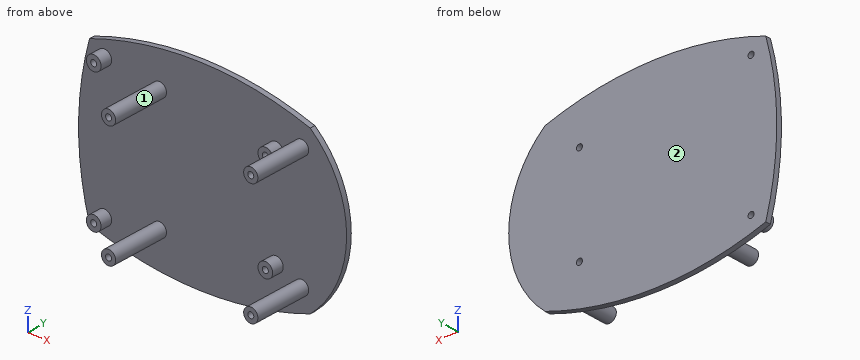
Autodesk Inventor part; units mm, degrees
ref_plane "Arbeitsebene1" through (41.47, 0, -24.5) normal (-0.3949, 0, -0.9187) x (0, -1, 0)
ref_plane "YZ Plane" through (0, 0, 0) normal (1, 0, 0) x (0, 1, 0)
ref_plane "XZ Plane" through (0, 0, 0) normal (0, 1, 0) x (-1, 0, 0)
sketch "Skizze4" plane through (0, 0, 0) normal (0, 1, 0) x (-1, 0, 0)
  arc A0 (45, -32.5) -> (45, 32.5) centre (-70.5152, 0) ccw
  arc A1 (45, 32.5) -> (-45, 32.5) centre (0, -98.75) ccw
  arc A2 (-45, 32.5) -> (-45, -32.5) centre (-16.8442, 0) ccw
  line L0 (49.4848, 0) -> (-59.8442, 0) construction
  circle A3 centre (39, -28) radius 1.225
  circle A4 centre (39, 28) radius 1.225
  circle A5 centre (-31, 20) radius 1.225
  circle A6 centre (-31, -20) radius 1.225
  circle A7 centre (16.53, -24.5) radius 1.225
  circle A8 centre (16.53, 24.5) radius 1.225
  circle A9 centre (-41.47, 24.5) radius 1.225
  circle A10 centre (-41.47, -24.5) radius 1.225
  line L1 (39, 28) -> (39, -28) construction
  line L2 (39, -28) -> (-31, -20) construction
  line L3 (-31, -20) -> (-31, 20) construction
  line L4 (-31, 20) -> (39, 28) construction
  line L5 (16.53, 24.5) -> (16.53, -24.5) construction
  line L6 (16.53, -24.5) -> (-41.47, -24.5) construction
  line L7 (-41.47, -24.5) -> (-41.47, 24.5) construction
  line L8 (-41.47, 24.5) -> (16.53, 24.5) construction
  line L9 (0, -40) -> (0, 40) construction
  circle A11 centre (16.53, -24.5) radius 2.9
  circle A12 centre (-41.47, -24.5) radius 2.9
  circle A13 centre (-41.47, 24.5) radius 2.9
  circle A14 centre (16.53, 24.5) radius 2.9
  line L10 (45, 32.5) -> (45, -32.5) construction
  line L11 (-45, 32.5) -> (-45, -32.5) construction
  arc A15 (-45, -32.5) -> (45, -32.5) centre (0, 98.75) ccw
  circle A16 centre (-31, -20) radius 3
  circle A17 centre (-31, 20) radius 3
  circle A18 centre (39, 28) radius 3
  circle A19 centre (39, -28) radius 3
  point P0 (0, 0)
  point P1 (0, 0)
  dimension "d19" = 2.45
  dimension "d20" = 5.8
  dimension "d28" = 80
  dimension "d30" = 90
  dimension "d31" = 58
  dimension "d32" = 49
  dimension "d33" = 56
  dimension "d34" = 40
  dimension "d35" = 70
  dimension "d36" = 65
  dimension "d37" = 65
  dimension "d38" = 22.47
  dimension "d39" = 120
  dimension "d40" = 6
  dimension "d41" = 2.45
  dimension "d42" = 43
  dimension "d58" = 6
sketch "Skizze3" plane through (0, 0, 0) normal (0, 1, 0) x (-1, 0, 0)
  line L0 (-220.6772, -144.4743) -> (-220.6772, -104.4743)
  line L1 (-220.6772, -104.4743) -> (-150.6772, -96.4743)
  line L2 (-150.6772, -96.4743) -> (-150.6772, -152.4743)
  line L3 (-150.6772, -152.4743) -> (-220.6772, -144.4743)
  line L4 (-173.154, -148.9743) -> (-231.154, -148.9743)
  line L5 (-231.154, -148.9743) -> (-231.154, -99.9743)
  line L6 (-231.154, -99.9743) -> (-173.154, -99.9743)
  line L7 (-173.154, -99.9743) -> (-173.154, -148.9743)
  circle A0 centre (-231.154, -99.9743) radius 1.35
  circle A1 centre (-231.154, -148.9743) radius 1.35
  circle A2 centre (-173.154, -148.9743) radius 1.35
  circle A3 centre (-173.154, -99.9743) radius 1.35
  arc A4 (-234.6505, -110.3469) -> (-234.6486, -138.3994) centre (-219.7787, -124.3722) ccw
  line L8 (-234.6505, -110.3469) -> (-234.6458, -99.4805)
  arc A5 (-231.5992, -96.4365) -> (-234.6458, -99.4805) centre (-231.6005, -99.4818) ccw
  line L9 (-231.5992, -96.4365) -> (-212.1876, -96.4449)
  arc A6 (-178.6836, -89.0505) -> (-212.1876, -96.4449) centre (-176.7514, -177.4047) ccw
  arc A7 (-149.827, -93.1805) -> (-178.6836, -89.0505) centre (-181.982, -214.9715) ccw
  arc A8 (-147.411, -95.6063) -> (-149.827, -93.1805) centre (-150.6924, -96.4584) ccw
  arc A9 (-143.2995, -124.3735) -> (-147.411, -95.6063) centre (-273.1451, -128.2544) ccw
  arc A10 (-147.4215, -153.3903) -> (-143.2995, -124.3735) centre (-273.1519, -120.7284) ccw
  arc A11 (-149.7866, -155.739) -> (-147.4215, -153.3903) centre (-150.6843, -152.4698) ccw
  arc A12 (-178.6402, -159.8288) -> (-149.7866, -155.739) centre (-181.7729, -33.9036) ccw
  arc A13 (-212.2336, -152.5079) -> (-178.6402, -159.8288) centre (-176.9785, -71.4691) ccw
  line L10 (-231.6452, -152.4995) -> (-212.2336, -152.5079)
  arc A14 (-234.6534, -149.2659) -> (-231.6452, -152.4995) centre (-231.6139, -149.4543) ccw
  line L11 (-234.6534, -149.2659) -> (-234.6486, -138.3994)
  line L12 (-240.2208, -124.3735) -> (-143.2995, -124.3735) construction
  line L13 (-177.3977, -89.0907) -> (-177.3977, -159.7918) construction
  point P0 (-177.3977, -124.4413)
extrude "Extrusion1" add sketch "Skizze4" along normal blind 2.2 contours A15 A2 A1 A0 | A7 | A8 | A9 | A10 | A11 | A12 | A13 | A14 | A16 | A17 | A18 | A19
extrude "Extrusion2" add sketch "Skizze4" against normal blind 24 contours A11 | A12 | A13 | A14
extrude "Extrusion3" add sketch "Skizze4" against normal blind 5 contours A16 | A17 | A18 | A19
ref_plane "Arbeitsebene1" through (41.47, 0, -24.5) normal (-0.3949, 0, -0.9187) x (0, -1, 0)
sketch "Skizze6" plane through (41.47, 0, -24.5) normal (-0.3949, 0, -0.9187) x (0, -1, 0)
  line L0 (24, 1.2564) -> (24.1406, 1.5)
  line L1 (24.1406, 1.5) -> (24.1969, 1.5)
  line L2 (24.1969, 1.5) -> (24.3375, 1.2564)
  line L3 (24.3375, 1.2564) -> (24.3937, 1.2564)
  line L4 (24.45, 1.2564) -> (24.45, 1.5487) construction
  line L5 (24.45, 1.5487) -> (23.8875, 1.5487) construction
  line L6 (23.8875, 1.5487) -> (23.8875, 1.2564) construction
  line L7 (23.8875, 1.2564) -> (23.9437, 1.2564) construction
  line L8 (23.9437, 1.2564) -> (24, 1.2564)
  line L9 (24.3937, 1.2564) -> (24.45, 1.2564) construction
  line L10 (24, 1.2564) -> (24.3375, 1.2564) construction
  line L11 (24.1406, 1.5) -> (24.1687, 1.5487) construction
  line L12 (24.1969, 1.5) -> (24.1687, 1.5487) construction
  line L13 (23.8875, 0) -> (24.45, 0) construction
  line L14 (23.8875, 1.2564) -> (23.9437, 1.159) construction
  line L15 (23.9437, 1.159) -> (24, 1.2564) construction
  line L16 (24.3375, 1.2564) -> (24.3937, 1.159) construction
  line L17 (24.3937, 1.159) -> (24.45, 1.2564) construction
  line L18 (24.1687, 1.2564) -> (24.1687, 1.5487) construction
  line L19 (23.9437, 1.159) -> (24.3937, 1.159) construction
  line L20 (23.8875, 0) -> (23.8875, 1.2564) construction
  line L21 (24.45, 0) -> (24.45, 1.2564) construction
  line L22 (-7.98, 0) -> (29.33, 0)
  line L23 (24, 1.225) -> (24, -1.225)
  line L24 (24, 1.2564) -> (24.3375, 1.2564)
  line L25 (-2.5375, 12.6525) -> (-2.3969, 12.8961)
  line L26 (-2.3969, 12.8961) -> (-2.3406, 12.8961)
  line L27 (-2.3406, 12.8961) -> (-2.2, 12.6525)
  line L28 (-2.2, 12.6525) -> (-2.1437, 12.6525)
  line L29 (-2.0875, 12.6525) -> (-2.0875, 12.9448) construction
  line L30 (-2.0875, 12.9448) -> (-2.65, 12.9448) construction
  line L31 (-2.65, 12.9448) -> (-2.65, 12.6525) construction
  line L32 (-2.65, 12.6525) -> (-2.5937, 12.6525) construction
  line L33 (-2.5937, 12.6525) -> (-2.5375, 12.6525)
  line L34 (-2.1437, 12.6525) -> (-2.0875, 12.6525) construction
  line L35 (-2.5375, 12.6525) -> (-2.2, 12.6525) construction
  line L36 (-2.3969, 12.8961) -> (-2.3687, 12.9448) construction
  line L37 (-2.3406, 12.8961) -> (-2.3687, 12.9448) construction
  line L38 (-2.65, 11.3961) -> (-2.0875, 11.3961) construction
  line L39 (-2.65, 12.6525) -> (-2.5937, 12.5551) construction
  line L40 (-2.5937, 12.5551) -> (-2.5375, 12.6525) construction
  line L41 (-2.2, 12.6525) -> (-2.1437, 12.5551) construction
  line L42 (-2.1437, 12.5551) -> (-2.0875, 12.6525) construction
  line L43 (-2.3687, 12.6525) -> (-2.3687, 12.9448) construction
  line L44 (-2.5937, 12.5551) -> (-2.1437, 12.5551) construction
  line L45 (-2.65, 11.3961) -> (-2.65, 12.6525) construction
  line L46 (-2.0875, 11.3961) -> (-2.0875, 12.6525) construction
  line L47 (29.33, 11.3961) -> (-7.98, 11.3961)
  line L48 (-2.5375, 12.6525) -> (-2.2, 12.6525)
  line L49 (-2.2, 10.1711) -> (-2.2, 12.6211)
  dimension "d47" = 60
  dimension "d48" = 3
  dimension "d49" = 0.45
  dimension "d50" = 2.5129
  dimension "d51" = 0.2436
  dimension "d52" = 0.0487
  dimension "d62" = 0
  dimension "d71" = 60
  dimension "d72" = 3
  dimension "d73" = 0.45
  dimension "d74" = 2.5129
  dimension "d75" = 0.2436
  dimension "d76" = 0.0487
  dimension "d82" = 0
equation "\"d53\" = 60deg"
equation "\"d54\" = 3"
equation "\"d55\" = 0.45"
equation "\"d56\" = 2.51288"
equation "\"d57\" = 0.3897"
equation "\"d77\" = 60deg"
equation "\"d78\" = 3"
equation "\"d79\" = 0.45"
equation "\"d80\" = 2.51288"
equation "\"d81\" = 0.3897"
properties part number "_3D-Druck"
The listing builds one solid part. Answer for the finished solid, in the listing's coordinates (mm). Face numbers are marked on the shaded views. Give positions to 0.01 mm unless a question says otherwise; leave off trailing zeros. Loops run counter-clockwise (first coordinate to the right, second up) from the corner with the lowest first, then second, coordinate; pieces in that order, holes last. Notation, with made-up numbers: (87.5, 29.5) - (93.5, 29.5) arc R20 cw to (93.5, 60.5) - close; hole circle Ø10 at (30.25, 76.5). An arc over 180 degrees is marked (long way). Use one line per item in the form item = value.
1. Section C-C on z = -20 is taken. Give the vertices of the cut face in (x, y) (3 decimals).
Calculated:
outline = (-47.806, 0) - (28, 0) - (28, -5) - (29.775, -5) - (29.775, 2.2) - (-47.806, 2.2) - close; (32.225, -5) - (34, -5) - (34, 0) - (54.91, 0) - (54.91, 2.2) - (32.225, 2.2) - close
2. Section B-B on x = -39 is taken. Give the vertices of the cut face in (y, z) (3 decimals).
Calculated:
outline = (-5, -31) - (0, -31) - (0, -34.406) - (2.2, -34.406) - (2.2, -29.225) - (-5, -29.225) - close; (-5, -26.775) - (2.2, -26.775) - (2.2, 26.775) - (-5, 26.775) - (-5, 25) - (0, 25) - (0, -25) - (-5, -25) - close; (-5, 29.225) - (2.2, 29.225) - (2.2, 34.406) - (0, 34.406) - (0, 31) - (-5, 31) - close
3. Section A-A on y = -19.75 is taken. Give the vertices of the cut face in (x, z) (3 decimals).
Calculated:
outline = circle Ø5.8 at (-16.53, -24.5); circle Ø5.8 at (-16.53, 24.5); circle Ø5.8 at (41.47, -24.5); circle Ø5.8 at (41.47, 24.5); hole circle Ø2.45 at (-16.53, -24.5); hole circle Ø2.45 at (-16.53, 24.5); hole circle Ø2.45 at (41.47, -24.5); hole circle Ø2.45 at (41.47, 24.5)
4. The mould has two halves that part along Z. Classify the marked faces 1 and 2: pulls with the +Z half, pulls with the -Z half, needs draft (parallel to the pull), parting line crosses it, or undercut.
Calculated:
face_1 = undercut
face_2 = needs draft
5. Find the intervals of material crossed by line 1 along Z through (x, y) = (31, -2.25) (3 decimals); line 2 along X through (y, z) = (-2.75, 24); line 3 along Z through (x, y) = (42.5, -14.75), in increasing order. Write a range as [from, to].
Calculated:
line_1 = [-23, -21.225], [-18.775, -17], [17, 18.775], [21.225, 23]
line_2 = [-19.39, -17.65], [-15.41, -13.67], [38.61, 40.35], [42.59, 44.33]
line_3 = [-27.21, -25.16], [-23.84, -21.79], [21.79, 23.84], [25.16, 27.21]
6. Given pin 1 Ø1.2 at (x, z) = (-16, -24.5) entering from -Y; pin 2 Ø3 at (x, z) = (-39, 28) entering from -Y; pin 3 Ø2 at (x, z) = (31, -20) entering from -Y; pin 4 Ø8 at (x, y) = (32, -3.5) entering from +Z, each flat-ended and moving along its own axis, determine where each tip first touches the part or whether it passes through.
Calculated:
pin_1 = 0
pin_2 = -5
pin_3 = through
pin_4 = 36.7
7. Section D-D on x = 41.47 is taken. Give the vertices of the cut face in (y, z) (3 decimals), then the cut area to 3 significant figures.
Calculated:
outline = (-24, -27.4) - (0, -27.4) - (0, -33.658) - (2.2, -33.658) - (2.2, 33.658) - (0, 33.658) - (0, 27.4) - (-24, 27.4) - (-24, 25.725) - (0, 25.725) - (0, 23.275) - (-24, 23.275) - (-24, 21.6) - (0, 21.6) - (0, -21.6) - (-24, -21.6) - (-24, -23.275) - (0, -23.275) - (0, -25.725) - (-24, -25.725) - close
area = 309 mm^2
